Build history of the part. All positions in model axes, mm. Face numbers are marked on the shaded views. A direction names the side the tool comes from. Round coordinates to 2 decimals unless told otherwise and drop trailing zeros. Order: outer loops, then holes, each group sorted by start corner. A loop starts at its lowest first (then second) coordinate and runs counter-clockwise, first axis right, second up. Notation, with made-up numbers: (81, -22.75) -> (122, -22.75) arc R29 ccw to (122, 14.25) -> close; hole circle Ø3 at (44, -38). An arc over 180 degrees is marked (long way). Answer as CSV lines item,"result". Start each with the question number.
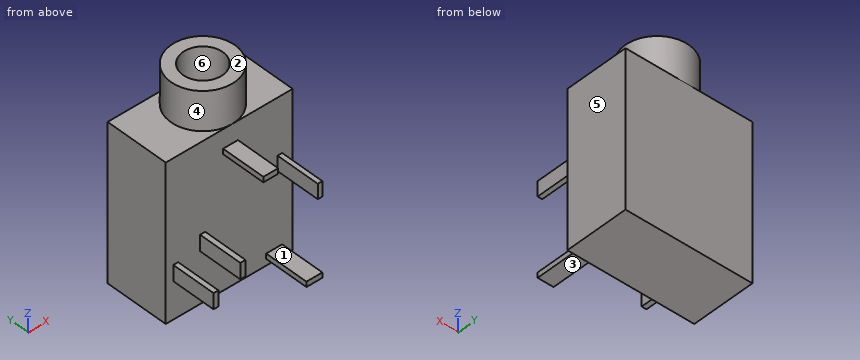
```python
from build123d import *

# Parameters (mm, degrees)
SKETCH_1_W      = 14.039038814
SKETCH_1_H      = 5.781099621
EXTRUDE_1_DEPTH = 5.75
SKETCH_2_R      = 2.89054981
SKETCH_2_R_2    = 1.8
EXTRUDE_2_DEPTH = 3.5
SKETCH_3_W      = 1.445545422
SKETCH_3_H      = 0.46914779
SKETCH_3_W_2    = 0.440036949
SKETCH_3_H_2    = 1.412750204
SKETCH_3_W_3    = 0.463196789
SKETCH_3_H_3    = 1.435910044
SKETCH_3_W_4    = 0.41687711
SKETCH_3_H_4    = 1.343270685
SKETCH_3_W_5    = 1.343270686
SKETCH_3_H_5    = 0.486356628
EXTRUDE_3_DEPTH = 4


with BuildPart() as part:
    # Эскиз1 → Бобышка-Вытянуть1 (new, symmetric)
    with BuildSketch(Plane(origin=(0, 0, 0), x_dir=(0, 0, -1), z_dir=(1, 0, 0))):
        with Locations((7.031108734, 2.884562427)):
            Rectangle(SKETCH_1_W, SKETCH_1_H)
    extrude(amount=EXTRUDE_1_DEPTH, both=True)

    # Эскиз2 → Бобышка-Вытянуть2 (add)
    with BuildSketch(Plane.XY.offset(-0.011589327)):
        with Locations(Location((0.25, 2.884562426, 0), (0, 0, 270))):
            Circle(SKETCH_2_R)
        with Locations((0.25, 2.884562426)):
            Circle(SKETCH_2_R_2, mode=Mode.SUBTRACT)
    extrude(amount=EXTRUDE_2_DEPTH)

    # Эскиз3 → Бобышка-Вытянуть3 (add)
    with BuildSketch(Plane.XZ.offset(0.005987384)):
        with Locations((4.077721902, -13.234721413)):
            Rectangle(SKETCH_3_W, SKETCH_3_H)
        with Locations((-4.845578503, -10.005870434)):
            Rectangle(SKETCH_3_W_2, SKETCH_3_H_2)
        with Locations((-2.402215445, -8.743659186)):
            Rectangle(SKETCH_3_W_3, SKETCH_3_H_3)
        with Locations((4.592056058, -5.732880063)):
            Rectangle(SKETCH_3_W_4, SKETCH_3_H_4)
        with Locations((0.122207051, -1.946246319)):
            Rectangle(SKETCH_3_W_5, SKETCH_3_H_5)
    extrude(amount=EXTRUDE_3_DEPTH)


solid = part.part
```
Q1. Slice it at D-D, the plane y = 1.5. Write the cut outline in (x, z).
Q2. Slice it at A-A, the plane y = -1.5. Write the cut outline in (x, z).
Q3. Which spindle directions (+Z, -Z, +X, -X, +Y, -Y) get a long thin tool onto all of the face, cutting with end or side? Do the marked faces 5 and 6. Say none if no direction does.
Q4. Two-plate mould, pull along Z, no slides. Class the marked faces 1, 2, 3 and 4: +Z half, -Z half, draft (parallel to the pull), parting line (faces both ways), or undercut.
Q5. Probe L1, parallel to Z at x = -4.5, y = 3.25; L2, parallel to X at y = -2.75, z = -5.25; L3, parallel to Z at x = -2.25, y = -3.5. List the from-to ranges inside material, lowest first.
Q6. Flat gauge pins, fed straight in: pin 1 Ø2 at (y, z) = (-3, 0.5) entering from -X; pin 2 Ø0.5 at (x, y) = (4.5, -2) entering from +Z; pin 3 Ø0.5 at (y, z) = (-2, -2) entering from +X; pin 4 Ø0.5 at (x, y) = (-2.5, -1.5) entering from +Z. Where does each tip first touch, or does it go through?
Q7. Slice it at C-C, the plane x = 1.5. Write the cut outline in (y, z), plus the area to 3 significant figures.
Q8. Slice it at B-B, the plane z = -5.5. Write the cut outline in (x, y), plus the area to 4 significant figures.
Solutions:
1,outline,"(-5.75, -14.05) -> (5.75, -14.05) -> (5.75, -0.01) -> (2.79, -0.01) -> (2.79, 3.49) -> (1.4, 3.49) -> (1.4, -0.01) -> (-0.9, -0.01) -> (-0.9, 3.49) -> (-2.29, 3.49) -> (-2.29, -0.01) -> (-5.75, -0.01) -> close"
2,outline,"(-5.07, -10.71) -> (-4.63, -10.71) -> (-4.63, -9.3) -> (-5.07, -9.3) -> close; (-2.63, -9.46) -> (-2.17, -9.46) -> (-2.17, -8.03) -> (-2.63, -8.03) -> close; (-0.55, -2.19) -> (0.79, -2.19) -> (0.79, -1.7) -> (-0.55, -1.7) -> close; (3.35, -13.47) -> (4.8, -13.47) -> (4.8, -13) -> (3.35, -13) -> close; (4.38, -6.4) -> (4.8, -6.4) -> (4.8, -5.06) -> (4.38, -5.06) -> close"
3,face 5,"+Z, -Z, +X, +Y, -Y"
3,face 6,"+Z"
4,face 1,"undercut"
4,face 2,"+Z half"
4,face 3,"-Z half"
4,face 4,"draft"
5,L1,"z = -14.05 to -0.01"
5,L2,"x = 4.38 to 4.8"
5,L3,"z = -9.46 to -8.03"
6,pin 1,"passes through"
6,pin 2,"stops at z = -5.06"
6,pin 3,"stops at x = 0.79"
6,pin 4,"stops at z = -8.03"
7,outline,"(-0.01, -14.05) -> (5.78, -14.05) -> (5.78, -0.01) -> (5.49, -0.01) -> (5.49, 3.49) -> (4.18, 3.49) -> (4.18, -0.01) -> (1.59, -0.01) -> (1.59, 3.49) -> (0.28, 3.49) -> (0.28, -0.01) -> (-0.01, -0.01) -> close"
7,area,"90.3 mm2"
8,outline,"(-5.75, -0.01) -> (4.38, -0.01) -> (4.38, -4.01) -> (4.8, -4.01) -> (4.8, -0.01) -> (5.75, -0.01) -> (5.75, 5.78) -> (-5.75, 5.78) -> close"
8,area,"68.15 mm2"
